Check sheet for the drawn part. Datum: minimum x, y, z corner. Units: mm. A direction names the side the tool comes from. Round coordinates to 2 decimals unless told otherwise and drop trailing zeros. Loops run counter-clockwise (first coordinate to the right, second up) from the corner with the lowest first, then second, coordinate; pieces in that order, holes last.
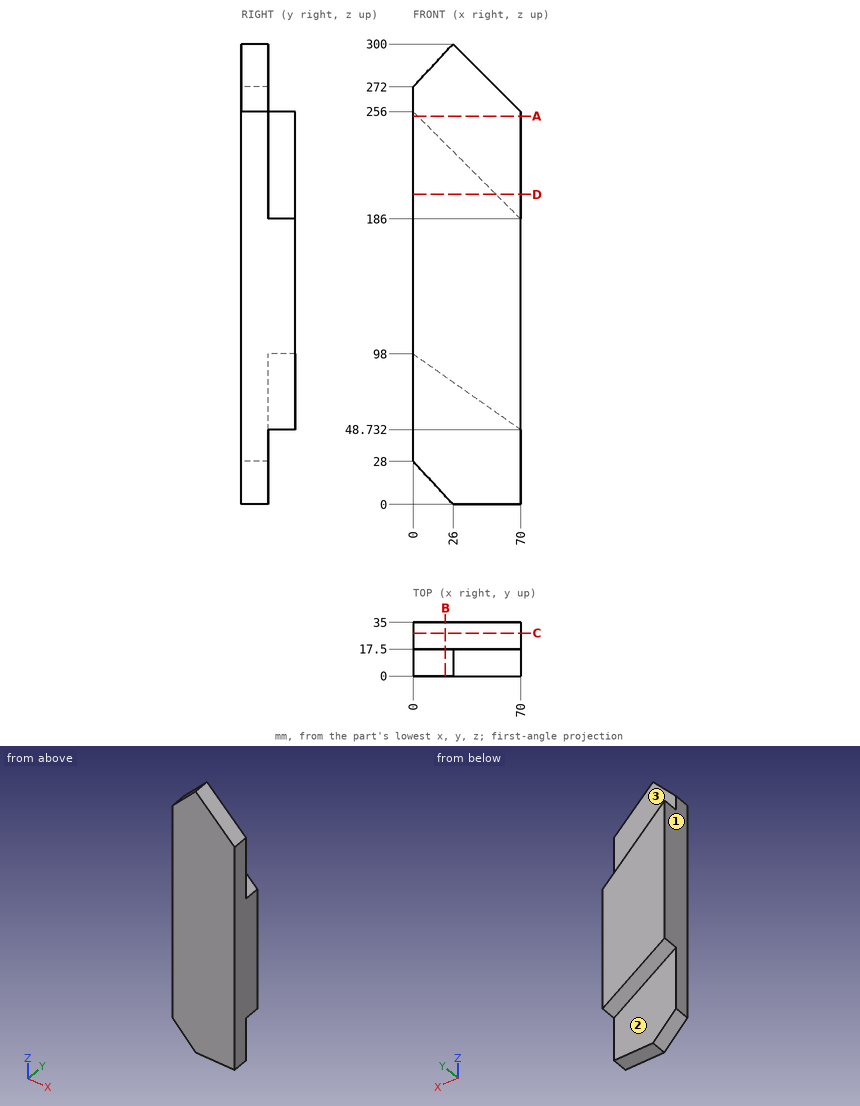
1) Sectioned sample at D-D, the plane z = 202. Record the cut outline in (x, y), then the cut area to 3 significant figures.
Report:
outline: (0, 0) - (70, 0) - (70, 17.5) - (54, 17.5) - (54, 35) - (0, 35) - close
area: 2,170 mm2
2) Sectioned sample at B-B, the plane x = 21. Record the cut outline in (y, z) (1 decimal), then the cut area to 3 significant figures.
Report:
outline: (0, 5.4) - (17.5, 5.4) - (17.5, 83.2) - (35, 83.2) - (35, 235) - (17.5, 235) - (17.5, 294.6) - (0, 294.6) - close
area: 7,720 mm2
3) Access from +Z, -Z, +X, -X, +Y, -Y to the whole of each face (thin tool, end or side, straight path). Record for the marked faces 1, 2 and 3.
Report:
face 1: +Z, -Z, -X, +Y, -Y
face 2: -Z, -X, +Y
face 3: +Z, +X, +Y
4) Sectioned sample at C-C, the plane y = 28. Record the cut outline in (x, z).
Report:
outline: (0, 98) - (70, 48.73) - (70, 186) - (0, 256) - close
5) Gauge pin test, flat ends, axial feed: pin 1 (8 mm diameter, centred on x = 41.5, y = 31, fed in from -Z) (1 decimal); pin 2 (5 mm diameter, centred on x = 35, y = 21, fed in from -Z); pin 3 (8 mm diameter, centred on x = 18.5, y = 25, fed in from -Z). Record the tip position at first contact, or that the pin passes through.
Report:
pin 1: stops at z = 66
pin 2: stops at z = 71.61
pin 3: stops at z = 82.16
6) Sectioned sample at A-A, the plane z = 253. Record the cut outline in (x, y), then the cut area to 3 significant figures.
Report:
outline: (0, 0) - (70, 0) - (70, 17.5) - (3, 17.5) - (3, 35) - (0, 35) - close
area: 1,280 mm2
7) Scan lines: line 1 along Y through (x, z) = (39.5, 248); line 2 along Z through (x, y) = (4, 10); line 3 along Z through (x, y) = (52, 31.5). Record each from-to range of solid material in increasing order.
Report:
line 1: y = 0 to 17.5
line 2: z = 23.69 to 276.31
line 3: z = 61.4 to 204
